```python
from build123d import *

# Parameters (mm, degrees)
ESQUISSE3_R                  = 14.8
BOSS_EXTRU_1_DEPTH           = 2
BOSS_EXTRU_2_REACH           = 31.138
R_P_TITION_CIRCULAIRE1_COUNT = 3
ENL_V_MAT_EXTRU_1_DEPTH      = 30.137604569
ENL_V_MAT_EXTRU_1_DEPTH_BACK = 30.137604569
ESQUISSE5_R                  = 1.625
BOSS_EXTRU_3_START           = 2
ESQUISSE6_R                  = 11
ESQUISSE6_R_2                = 1.625
BOSS_EXTRU_3_DEPTH           = 2


with BuildPart() as part:
    # Esquisse2 → Révolution1 (revolve)
    with BuildSketch(Plane(origin=(0, 0, 0), x_dir=(0, 0, -1), z_dir=(1, 0, 0)), mode=Mode.PRIVATE) as r_volution1_sk:
        Polygon((0, 0), (0, 20), (5, 15), (5, 0), align=None)
    revolve(r_volution1_sk.sketch.rotate(Axis((0, 0, 0), (0, 0, -1)), 90), axis=Axis((0, 0, 0), (0, 0, -1)))

    # Esquisse3 → Boss.-Extru.1 (add)
    with BuildSketch(Plane(origin=(0, 0, -5), x_dir=(-1, 0, 0), z_dir=(0, 0, -1))):
        Circle(ESQUISSE3_R)
    extrude(amount=BOSS_EXTRU_1_DEPTH)

    # Boss.-Extru.2: up to this face of the body (flat: up to its plane)
    boss_extru_2_end = Plane(part.part.faces().sort_by_distance((0, 0, -7))[0])
    # Esquisse4 → Boss.-Extru.2 (add, up to the picked face)
    with BuildSketch(Plane.XY, mode=Mode.PRIVATE) as boss_extru_2_sk1:
        with BuildLine():
            Line((1.5, 19.943670675), (-1.5, 19.943670675))
            Line((-1.5, 19.943670675), (-3.52737474, 14.373504355))
            ThreePointArc((-3.52737474, 14.373504355), (0, 14.8), (3.52737474, 14.373504355))
            Line((3.52737474, 14.373504355), (1.5, 19.943670675))
        make_face()
    boss_extru_2_tool1 = split(extrude(boss_extru_2_sk1.sketch, amount=-BOSS_EXTRU_2_REACH, mode=Mode.PRIVATE), bisect_by=boss_extru_2_end, keep=Keep.BOTH, mode=Mode.PRIVATE)
    boss_extru_2 = boss_extru_2_tool1.solids().sort_by(Axis((0, 16.957577, 0), (0, 0, -1)))[0]
    add(boss_extru_2)

    # Répétition circulaire1: Boss.-Extru.2 ×3 about axis
    r_p_tition_circulaire1_axis = Axis((0, 0, 0), (0, 0, 1))
    for i in range(1, R_P_TITION_CIRCULAIRE1_COUNT):
        add(boss_extru_2.rotate(r_p_tition_circulaire1_axis, i * 360 / R_P_TITION_CIRCULAIRE1_COUNT))

    # Esquisse5 → Enlèv. mat.-Extru.1 (cut, two sides: drawn at the far end of the back side and taken through both)
    with BuildSketch(Plane.XY.offset(-ENL_V_MAT_EXTRU_1_DEPTH_BACK)):
        with Locations((0, 7)):
            Circle(ESQUISSE5_R)
        Circle(ESQUISSE5_R)
        with Locations((7, 0)):
            Circle(ESQUISSE5_R)
        with Locations((0, -7)):
            Circle(ESQUISSE5_R)
        with Locations((-7, 0)):
            Circle(ESQUISSE5_R)
    extrude(amount=ENL_V_MAT_EXTRU_1_DEPTH + ENL_V_MAT_EXTRU_1_DEPTH_BACK, mode=Mode.SUBTRACT)

    # Esquisse6 → Boss.-Extru.3 (add)
    with BuildSketch(Plane.XY.offset(BOSS_EXTRU_3_START)):
        with Locations(Location((0, 0, 0), (0, 0, 180))):
            Circle(ESQUISSE6_R)
        with Locations((0, 7)):
            Circle(ESQUISSE6_R_2, mode=Mode.SUBTRACT)
        with Locations((0, -7)):
            Circle(ESQUISSE6_R_2, mode=Mode.SUBTRACT)
        Circle(ESQUISSE6_R_2, mode=Mode.SUBTRACT)
        with Locations((7, 0)):
            Circle(ESQUISSE6_R_2, mode=Mode.SUBTRACT)
        with Locations((-7, 0)):
            Circle(ESQUISSE6_R_2, mode=Mode.SUBTRACT)
    extrude(amount=-BOSS_EXTRU_3_DEPTH)


solid = part.part
```
Source: CAD feature listing. Evaluate the final solid. Frame: model axes, mm. A direction names the side the tool comes from. Coordinates: 2 decimals unless noted, no trailing zeros. Write each loop counter-clockwise with the first axis right and the second up, starting at its lowest first coordinate (ties: lowest second). Pieces come first, ordered by that corner, then holes. Notation, with made-up numbers: (-37.75, -22.75) - (-30.75, -22.75) arc R19 ccw to (-30.75, 11.25) - close; hole circle Ø6 at (-9, -22.5). An arc over 180 degrees is marked (long way). Answer as a JSON object with one key per item and string values.
Q1. Section query C-C, the plane z = -3. Output: boundary loops of the cut face in (x, y) (3 decimals).
Ans:
{"outline": "(-18.022, -8.673) - (-16.522, -11.271) - (-13.219, -10.689) arc R17 ccw to (13.219, -10.689) - (16.522, -11.271) - (18.022, -8.673) - (15.866, -6.104) arc R17 ccw to (2.647, 16.793) - (1.5, 19.944) - (-1.5, 19.944) - (-2.647, 16.793) arc R17 ccw to (-15.866, -6.104) - close; hole circle Ø3.25 at (-7, 0); hole circle Ø3.25 at (0, -7); hole circle Ø3.25 at (0, 0); hole circle Ø3.25 at (0, 7); hole circle Ø3.25 at (7, 0)"}
Q2. Material intervals for line 1 (Y direction, x = 0, z = 1.4) (3 decimals); line 2 (X direction, y = 0, z = -3) (3 decimals); line 3 (Y direction, x = 0, z = -1.75) (3 decimals), sorted ascending. Write a range as [from, to].
Ans:
{"line 1": "y = [-11, -8.625], [-5.375, -1.625], [1.625, 5.375], [8.625, 11]", "line 2": "x = [-17, -8.625], [-5.375, -1.625], [1.625, 5.375], [8.625, 17]", "line 3": "y = [-18.25, -8.625], [-5.375, -1.625], [1.625, 5.375], [8.625, 19.944]"}
Q3. Draft query along Y for faces 1 (the flat face through (14.211, -10.863, -4.229)), 2 (the cylindrical face through (12.733, 7.544, -5.986)), 3 (the cylindrical face through (2.38, 10.74, 1.01)). Return one class per face: released by +Y, released by -Y, zero draft, split by the parting line, or undercut.
Ans:
{"face 1": "released by -Y", "face 2": "undercut", "face 3": "split by the parting line"}
Q4. Section query B-B, the plane z = -5.75. State how many separate pieces and enclosed holes the cut face has, plus the area to 3 significant figures.
Ans:
{"separate pieces": "1", "enclosed holes": "5", "area": "725 mm2"}
Q5. First-contact query: pin 1 Ø3 at (x, z) = (-12, -2.5) entering from -Y; pin 2 Ø4 at (x, z) = (15.5, -4) entering from +Y; pin 3 Ø5 at (y, z) = (7, -1) entering from +X; pin 4 Ø1.9 at (x, y) = (0, -7) entering from +Z. Flat tips, straight axial feed; report the tip coordinate or a pass-through.
Ans:
{"pin 1": "stops at y = -15.06", "pin 2": "stops at y = 10.26", "pin 3": "stops at x = 19.44", "pin 4": "passes through"}
Q6. Set-up query: faces 4 (the flat face through (17.26, -9.99, -3.45)), 5 (the flat face through (2.3, 17.74, -4.23)), 6 (the flat face through (-9, 9, 0)), 7 (the flat face through (-17.282, -9.954, -3.451)), 8 (the flat face through (-16.513, -6.875, -4.229)). Return all of +Z, -Z, +X, -X, +Y, -Y with unobstructed straight access to the full face (end or side cutting, diameter ignored); none if empty.
Ans:
{"face 4": "-Z, +X, -Y", "face 5": "-Z, +X, +Y", "face 6": "+Z", "face 7": "-Z, -X, -Y", "face 8": "-Z, -X"}
Q7. Section query A-A, the plane x = 0. Output: boundary loops of the cut face in (y, z) (3 decimals).
Ans:
{"outline": "(-20, 0) - (-15, -5) - (-14.8, -5) - (-14.8, -7) - (-8.625, -7) - (-8.625, 2) - (-11, 2) - (-11, 0) - close; (-5.375, -7) - (-1.625, -7) - (-1.625, 2) - (-5.375, 2) - close; (1.625, -7) - (5.375, -7) - (5.375, 2) - (1.625, 2) - close; (8.625, -7) - (19.944, -7) - (19.944, -0.056) - (20, 0) - (11, 0) - (11, 2) - (8.625, 2) - close"}
